The listing builds one solid part. Answer for the finished solid, in the listing's coordinates (mm). Round coordinates to 2 decimals unless told otherwise and drop trailing zeros. Loops run counter-clockwise (first coordinate to the right, second up) from the corner with the lowest first, then second, coordinate; pieces in that order, holes last. Notation, with made-up numbers: (64, 3.25) - (74, 3.25) arc R16 cw to (74, 10.25) - close; hole circle Ø2 at (41.25, -38.75). An arc over 180 degrees is marked (long way). One line per question, with ' | ' between items. Start each with the question number.
from build123d import *

# Parameters (mm, degrees)
F1_DEPTH = 0.05


with BuildPart() as f1:
    # F0 (on Front) → F1 (new body, symmetric)
    with BuildSketch(Plane.XZ):
        with BuildLine():
            ThreePointArc((-2.690905, 6.876757), (-2.692458, 6.77403), (-2.765534, 6.701815))
            ThreePointArc((-2.765534, 6.701815), (-2.774455, 6.698127), (-2.783371, 6.694427))
            ThreePointArc((-2.783371, 6.694427), (-2.886107, 6.693818), (-2.959844, 6.765359))
            Line((-2.959844, 6.765359), (-9.441598, 21.580797))
            ThreePointArc((-9.441598, 21.580797), (-10.179713, 22.775744), (-11.221047, 23.71826))
            ThreePointArc((-11.221047, 23.71826), (-22.627417, 22.627417), (-23.71826, 11.221047))
            ThreePointArc((-23.71826, 11.221047), (-22.775744, 10.179713), (-21.580797, 9.441598))
            Line((-21.580797, 9.441598), (-6.765359, 2.959844))
            ThreePointArc((-6.765359, 2.959844), (-6.693818, 2.886107), (-6.694427, 2.783371))
            ThreePointArc((-6.694427, 2.783371), (-6.698127, 2.774455), (-6.701815, 2.765534))
            ThreePointArc((-6.701815, 2.765534), (-6.77403, 2.692458), (-6.876757, 2.690905))
            Line((-6.876757, 2.690905), (-21.936146, 8.583709))
            ThreePointArc((-21.936146, 8.583709), (-23.303027, 8.906739), (-24.705821, 8.836865))
            ThreePointArc((-24.705821, 8.836865), (-32, 0), (-24.705821, -8.836865))
            ThreePointArc((-24.705821, -8.836865), (-23.303027, -8.906739), (-21.936146, -8.583709))
            Line((-21.936146, -8.583709), (-6.876757, -2.690905))
            ThreePointArc((-6.876757, -2.690905), (-6.77403, -2.692458), (-6.701815, -2.765534))
            ThreePointArc((-6.701815, -2.765534), (-6.698127, -2.774455), (-6.694427, -2.783371))
            ThreePointArc((-6.694427, -2.783371), (-6.693818, -2.886107), (-6.765359, -2.959844))
            Line((-6.765359, -2.959844), (-21.580797, -9.441598))
            ThreePointArc((-21.580797, -9.441598), (-22.775744, -10.179713), (-23.71826, -11.221047))
            ThreePointArc((-23.71826, -11.221047), (-22.627417, -22.627417), (-11.221047, -23.71826))
            ThreePointArc((-11.221047, -23.71826), (-10.179713, -22.775744), (-9.441598, -21.580797))
            Line((-9.441598, -21.580797), (-2.959844, -6.765359))
            ThreePointArc((-2.959844, -6.765359), (-2.886107, -6.693818), (-2.783371, -6.694427))
            ThreePointArc((-2.783371, -6.694427), (-2.774455, -6.698127), (-2.765534, -6.701815))
            ThreePointArc((-2.765534, -6.701815), (-2.692458, -6.77403), (-2.690905, -6.876757))
            Line((-2.690905, -6.876757), (-8.583709, -21.936146))
            ThreePointArc((-8.583709, -21.936146), (-8.906739, -23.303027), (-8.836865, -24.705821))
            ThreePointArc((-8.836865, -24.705821), (0, -32), (8.836865, -24.705821))
            ThreePointArc((8.836865, -24.705821), (8.906739, -23.303027), (8.583709, -21.936146))
            Line((8.583709, -21.936146), (2.690905, -6.876757))
            ThreePointArc((2.690905, -6.876757), (2.692458, -6.77403), (2.765534, -6.701815))
            ThreePointArc((2.765534, -6.701815), (2.774455, -6.698127), (2.783371, -6.694427))
            ThreePointArc((2.783371, -6.694427), (2.886107, -6.693818), (2.959844, -6.765359))
            Line((2.959844, -6.765359), (9.441598, -21.580797))
            ThreePointArc((9.441598, -21.580797), (10.179713, -22.775744), (11.221047, -23.71826))
            ThreePointArc((11.221047, -23.71826), (22.627417, -22.627417), (23.71826, -11.221047))
            ThreePointArc((23.71826, -11.221047), (22.775744, -10.179713), (21.580797, -9.441598))
            Line((21.580797, -9.441598), (6.765359, -2.959844))
            ThreePointArc((6.765359, -2.959844), (6.693818, -2.886107), (6.694427, -2.783371))
            ThreePointArc((6.694427, -2.783371), (6.698127, -2.774455), (6.701815, -2.765534))
            ThreePointArc((6.701815, -2.765534), (6.77403, -2.692458), (6.876757, -2.690905))
            Line((6.876757, -2.690905), (21.936146, -8.583709))
            ThreePointArc((21.936146, -8.583709), (23.303027, -8.906739), (24.705821, -8.836865))
            ThreePointArc((24.705821, -8.836865), (32, 0), (24.705821, 8.836865))
            ThreePointArc((24.705821, 8.836865), (23.303027, 8.906739), (21.936146, 8.583709))
            Line((21.936146, 8.583709), (6.876757, 2.690905))
            ThreePointArc((6.876757, 2.690905), (6.77403, 2.692458), (6.701815, 2.765534))
            ThreePointArc((6.701815, 2.765534), (6.698127, 2.774455), (6.694427, 2.783371))
            ThreePointArc((6.694427, 2.783371), (6.693818, 2.886107), (6.765359, 2.959844))
            Line((6.765359, 2.959844), (21.580797, 9.441598))
            ThreePointArc((21.580797, 9.441598), (22.775744, 10.179713), (23.71826, 11.221047))
            ThreePointArc((23.71826, 11.221047), (22.627417, 22.627417), (11.221047, 23.71826))
            ThreePointArc((11.221047, 23.71826), (10.179713, 22.775744), (9.441598, 21.580797))
            Line((9.441598, 21.580797), (2.959844, 6.765359))
            ThreePointArc((2.959844, 6.765359), (2.886107, 6.693818), (2.783371, 6.694427))
            ThreePointArc((2.783371, 6.694427), (2.774455, 6.698127), (2.765534, 6.701815))
            ThreePointArc((2.765534, 6.701815), (2.692458, 6.77403), (2.690905, 6.876757))
            Line((2.690905, 6.876757), (8.583709, 21.936146))
            ThreePointArc((8.583709, 21.936146), (8.906739, 23.303027), (8.836865, 24.705821))
            ThreePointArc((8.836865, 24.705821), (0, 32), (-8.836865, 24.705821))
            ThreePointArc((-8.836865, 24.705821), (-8.906739, 23.303027), (-8.583709, 21.936146))
            Line((-8.583709, 21.936146), (-2.690905, 6.876757))
        make_face()
        with BuildLine():
            ThreePointArc((1.147858, 2.933415), (2.601754, 1.775774), (3.15, 0))
            ThreePointArc((3.15, 0), (-2.601754, -1.775774), (1.147858, 2.933415))
        make_face(mode=Mode.SUBTRACT)
    extrude(amount=F1_DEPTH, both=True)


solid = f1.part
(1) Find section B-B on z = 12.5. Write down the section's boundary in (x, y), plus the area to 3 significant figures.
(2) Consider L1, parallel to Z at x = 0, y = 0; L2, parallel to X at y = 0, z = -13.5; L3, parallel to X at y = 0, z = -19.5. Determine where each line is inside the solid, lowest interval first.
(3) Find section C-C on x = -20. Write down the section's boundary in (y, z).
(4) Find section A-A on x = 0. Write down the section's boundary in (y, z), plus the area to 3 significant figures.
Answer below:
1) outline: (-24.44, -0.05) - (-5.47, -0.05) - (-5.47, 0.05) - (-24.44, 0.05) - close; (-4.89, -0.05) - (4.89, -0.05) - (4.89, 0.05) - (-4.89, 0.05) - close; (5.47, -0.05) - (24.44, -0.05) - (24.44, 0.05) - (5.47, 0.05) - close | area: 4.77 mm2
2) L1: -32 to -3.15, 3.15 to 32 | L2: -24.83 to -5.91, -5.28 to 5.28, 5.91 to 24.83 | L3: -24.66 to -8.53, -7.63 to 7.63, 8.53 to 24.66
3) outline: (-0.05, -24.45) - (0.05, -24.45) - (0.05, -8.75) - (-0.05, -8.75) - close; (-0.05, -7.83) - (0.05, -7.83) - (0.05, 7.83) - (-0.05, 7.83) - close; (-0.05, 8.75) - (0.05, 8.75) - (0.05, 24.45) - (-0.05, 24.45) - close
4) outline: (-0.05, -32) - (0.05, -32) - (0.05, -3.15) - (-0.05, -3.15) - close; (-0.05, 3.15) - (0.05, 3.15) - (0.05, 32) - (-0.05, 32) - close | area: 5.77 mm2
